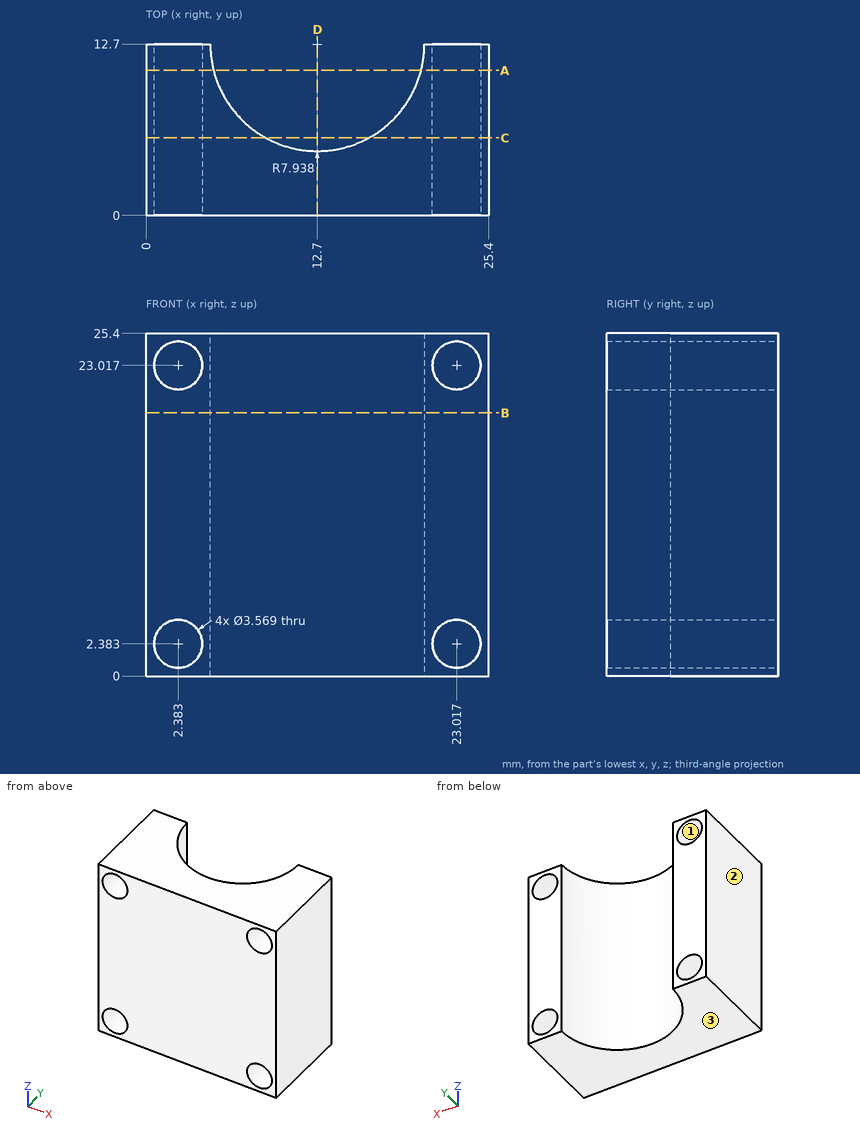
Check sheet for the drawn part. Datum: minimum x, y, z corner. Units: mm. Give positions to 0.01 mm unless a question says otherwise; leave off trailing zeros. Order: outer loops, then holes, each group sorted by start corner. A loop starts at its lowest first (then second) coordinate and runs counter-clockwise, first axis right, second up.
1. Draft check along X on the marked faces 1, 2 and 3. Enter one of: pulls with the +X half, pulls with the -X half, needs draft (parallel to the pull), parting line crosses it, or undercut.
Completed:
face 1: undercut
face 2: pulls with the -X half
face 3: needs draft
2. Scan lines: line 1 (X direction, y = 3, z = 2.5); line 2 (X direction, y = 11.75, z = 22.75); line 3 (Z direction, x = 24, y = 3.75) (1 decimal). Record each from-to range of solid material in increasing order.
Completed:
line 1: x = 0 to 0.6, 4.16 to 21.24, 24.8 to 25.4
line 2: x = 0 to 0.62, 4.15 to 4.82, 20.58 to 21.25, 24.78 to 25.4
line 3: z = 0 to 0.9, 3.9 to 21.5, 24.5 to 25.4
3. Sectioned sample at B-B (z = 19.5). Record the boundary of the cut face in (x, y) (1 decimal).
Completed:
outline: (0, 0) - (25.4, 0) - (25.4, 12.7) - (20.6, 12.7) arc R7.9 cw to (4.8, 12.7) - (0, 12.7) - close
4. Sectioned sample at D-D (x = 12.7). Record the boundary of the cut face in (y, z), then the cut area to 3 significant figures.
Completed:
outline: (0, 0) - (4.76, 0) - (4.76, 25.4) - (0, 25.4) - close
area: 121 mm2
5. Depth check by flat-ended pin: pin 1 (1 mm diameter, centred on x = 3, z = 3, fed in from -Y). Enter the tip coordinate at first touch or a pass-through.
Completed:
pin 1: passes through
6. Sectioned sample at C-C (y = 5.75). Record the boundary of the cut face in (x, z) (1 decimal).
Completed:
outline: (0, 0) - (8.9, 0) - (8.9, 25.4) - (0, 25.4) - close; (16.5, 0) - (25.4, 0) - (25.4, 25.4) - (16.5, 25.4) - close; hole circle Ø3.6 at (2.4, 2.4); hole circle Ø3.6 at (2.4, 23); hole circle Ø3.6 at (23, 2.4); hole circle Ø3.6 at (23, 23)
7. Sectioned sample at A-A (y = 10.75). Record the boundary of the cut face in (x, z) (1 decimal).
Completed:
outline: (0, 0) - (5, 0) - (5, 25.4) - (0, 25.4) - close; (20.4, 0) - (25.4, 0) - (25.4, 25.4) - (20.4, 25.4) - close; hole circle Ø3.6 at (2.4, 2.4); hole circle Ø3.6 at (2.4, 23); hole circle Ø3.6 at (23, 2.4); hole circle Ø3.6 at (23, 23)
